Design review of the part built by this model. Coordinates are the model's own, in mm. A direction names the side the tool comes from. Give positions to 0.01 mm unless a question says otherwise; leave off trailing zeros. Order: outer loops, then holes, each group sorted by start corner. A loop starts at its lowest first (then second) coordinate and runs counter-clockwise, first axis right, second up.
```python
from build123d import *

# Parameters (mm, degrees)
F1_DEPTH  = 22.5
F3_DEPTH  = 45
F4_R      = 4.3
F5_DEPTH  = 38.501
F6_W      = 39
F6_H      = 20.5
F7_DEPTH  = 18
F8_DEPTH  = 18
F9_R      = 4.3
F10_DEPTH = 3


with BuildPart() as f1:
    # F0 (on Right) → F1 (new body, symmetric)
    with BuildSketch(Plane.YZ):
        Polygon((0, 0), (40, 0), (40, 5), (-5, 5), (-5, -7.571068), (20.928932, -33.5), (53, -33.5), (53, -28.5), (23, -28.5), (0, -5.5), align=None)
    extrude(amount=F1_DEPTH, both=True)

    # F2 (on face) → F3 (join, through all)
    with BuildSketch(Plane.YZ.offset(22.5)):
        Polygon((-5, -7.571068), (-5, 5), (-23, 5), (-23, -33.5), (20.928932, -33.5), align=None)
    extrude(amount=-F3_DEPTH)

    # F4 (on face) → F5 (cut, through all)
    with BuildSketch(Plane.XY.offset(5)):
        with Locations((0, -14)):
            Circle(F4_R)
        with Locations((13.5, -14)):
            Circle(F4_R)
        with Locations((-13.5, -14)):
            Circle(F4_R)
    extrude(amount=-F5_DEPTH, mode=Mode.SUBTRACT)

    # F6 (on face) → F7 (cut)
    with BuildSketch(Plane.XZ.offset(23)):
        with Locations((0, -8.25)):
            Rectangle(F6_W, F6_H)
    extrude(amount=-F7_DEPTH, mode=Mode.SUBTRACT)

    # F6 (on face) → F8 (cut)
    with BuildSketch(Plane.XZ.offset(23)):
        with Locations((0, -8.25)):
            Rectangle(F6_W, F6_H)
    extrude(amount=-F8_DEPTH, mode=Mode.SUBTRACT)

    # F9 (on face) → F10 (join, through all)
    with BuildSketch(Plane.XY.offset(5)):
        with Locations((-13.5, -14)):
            Circle(F9_R)
        with Locations((0, -14)):
            Circle(F9_R)
        with Locations((13.5, -14)):
            Circle(F9_R)
    extrude(amount=-F10_DEPTH)


solid = f1.part
```
1. For pin 1 (6 mm diameter, centred on x = -6, z = -2.5, fed in from +Y); pin 2 (7 mm diameter, centred on x = 0, y = -14, fed in from -Z); pin 3 (1 mm diameter, centred on x = 4, z = -13.5, fed in from -Y), all flat-tipped, find the tip position at first contact; note any pin that passes through.
Recorded:
pin 1: stops at y = 40
pin 2: stops at z = 2
pin 3: stops at y = -5
2. For line 1 along Z through (x, y) = (-11, 34); line 2 along Y through (x, z) = (-13.5, -29.75); line 3 along Z through (x, y) = (-11.5, 43), list the stretches that pass through material, from the lowest coordinate up.
Recorded:
line 1: z = -33.5 to -28.5, 0 to 5
line 2: y = -23 to -18.3, -9.7 to 53
line 3: z = -33.5 to -28.5
3. Take a section at B-B (x = 0). State the section outline as (y, z) points.
Recorded:
outline: (-23, -33.5) - (-18.3, -33.5) - (-18.3, -18.5) - (-23, -18.5) - close; (-23, 2) - (-5, 2) - (-5, -18.5) - (-9.7, -18.5) - (-9.7, -33.5) - (53, -33.5) - (53, -28.5) - (23, -28.5) - (0, -5.5) - (0, 0) - (40, 0) - (40, 5) - (-23, 5) - close
4. Take a section at A-A (y = 37). State the section outline as (x, z) points, then the cut area to 3 significant figures.
Recorded:
outline: (-22.5, -33.5) - (22.5, -33.5) - (22.5, -28.5) - (-22.5, -28.5) - close; (-22.5, 0) - (22.5, 0) - (22.5, 5) - (-22.5, 5) - close
area: 450 mm2
5. Machinability: for faces 1 (the face through (-0.56, -9.737, -25.895)), 2 (the face through (0, 40, 2)), 3 (the face through (-22.5, -2, -14)), 4 (the face through (0, 38, -28.5)), 5 (the face through (-19.5, -14, -8)), which of the approach directions +Z, -Z, +X, -X, +Y, -Y give a long, thin tool a straight path to every point of the face, cutting with its end or side? Answer none if there is none.
Recorded:
face 1: -Z
face 2: +Z, +X, -X, +Y
face 3: +Z, -Z, -X, +Y, -Y
face 4: +X, -X, +Y
face 5: -Y
6. Take a section at D-D (z = -1). State the section outline as (x, y) points.
Recorded:
outline: (-22.5, -23) - (-19.5, -23) - (-19.5, -5) - (19.5, -5) - (19.5, -23) - (22.5, -23) - (22.5, 0) - (-22.5, 0) - close
7. Draft analysis for pull direction Z (two halves, no side actions). For faces 6 (the face through (0.3, 11.7, -17.2)), 7 (the face through (0, 9, 5)), 8 (the face through (19.5, -14, -8)), 9 (the face through (12.94, -9.737, -25.895)), state which applies: pulls with the +Z half, pulls with the -Z half, needs draft (parallel to the pull), parting line crosses it, or undercut.
Recorded:
face 6: undercut
face 7: pulls with the +Z half
face 8: undercut
face 9: needs draft
8. Take a section at C-C (y = -14). State the section outline as (x, z) points, then the cut area to 3 significant figures.
Recorded:
outline: (-22.5, -33.5) - (-17.8, -33.5) - (-17.8, -18.5) - (-19.5, -18.5) - (-19.5, 2) - (19.5, 2) - (19.5, -18.5) - (17.8, -18.5) - (17.8, -33.5) - (22.5, -33.5) - (22.5, 5) - (-22.5, 5) - close; (-9.2, -33.5) - (-4.3, -33.5) - (-4.3, -18.5) - (-9.2, -18.5) - close; (4.3, -33.5) - (9.2, -33.5) - (9.2, -18.5) - (4.3, -18.5) - close
area: 546 mm2
